```python
from build123d import *

# Parameters (mm, degrees)
F1_DEPTH       = 12
F3_D           = 5.5
F3_CSINK_D     = 12
F3_CSINK_ANGLE = 90


with BuildPart() as f1:
    # F0 (on Top) → F1 (new body)
    with BuildSketch(Plane.XY):
        with BuildLine():
            ThreePointArc((-17, 13.96424), (20.712315, -7.416198), (-22, 0))
            Line((-22, 0), (-22, 32.5))
            Line((-22, 32.5), (-32.5, 32.5))
            Line((-32.5, 32.5), (-32.5, 0))
            ThreePointArc((-32.5, 0), (-22.98097, -22.98097), (0, -32.5))
            Line((0, -32.5), (32.5, -32.5))
            Line((32.5, -32.5), (32.5, 32.5))
            Line((32.5, 32.5), (0, 32.5))
            Line((0, 32.5), (-17, 32.5))
            Line((-17, 32.5), (-17, 13.96424))
        make_face()
    extrude(amount=F1_DEPTH)

    # F3 (through all)
    with Locations(Plane(origin=(-32.5, 0, 0), x_dir=(0, -1, 0), z_dir=(-1, 0, 0))):
        with Locations((-26.5, 6)):
            CounterSinkHole(F3_D / 2, F3_CSINK_D / 2, counter_sink_angle=F3_CSINK_ANGLE)


solid = f1.part
```
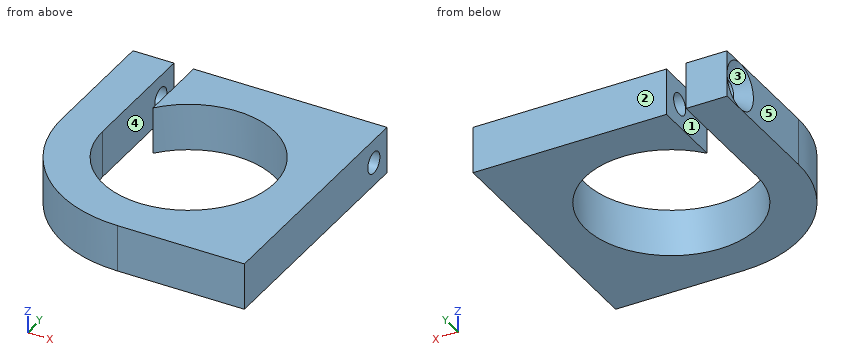
Read the model definition and answer for the solid it produces. Units are mm, in the model's axes. Face numbers are marked on the shaded views. A direction names the side the tool comes from. Coordinates: 2 decimals unless noted, no trailing zeros. Write each loop counter-clockwise with the first axis right and the second up, starting at its lowest first coordinate (ties: lowest second). Pieces come first, ordered by that corner, then holes. Notation, with made-up numbers: (-33.75, -8) -> (-28.75, -8) arc R17 ccw to (-28.75, 10) -> close; hole circle Ø10 at (71, -15). An arc over 180 degrees is marked (long way). Answer as a JSON object with one key per item and string values.
Q1. The part is cut by section B-B on y = 1.5. Give the vertices of the cut face in (x, z).
The answers:
{"outline": "(-32.5, 0) -> (-22, 0) -> (-22, 12) -> (-32.5, 12) -> close; (21.95, 0) -> (32.5, 0) -> (32.5, 12) -> (21.95, 12) -> close"}
Q2. Consider line 1 (Y direction, x = 0, z = 6.5); line 2 (Y direction, x = -1.5, z = 5.75); line 3 (Z direction, x = 1.5, y = 26.5). Determine where each line is inside the solid, lowest interval first. Write a range as [from, to].
The answers:
{"line 1": "y = [-32.5, -22], [22, 23.8], [29.2, 32.5]", "line 2": "y = [-32.47, -21.95], [21.95, 23.76], [29.24, 32.5]", "line 3": "z = [0, 3.25], [8.75, 12]"}
Q3. Determine the mould class of the marked faces 1, 2 and 3 for opening direction Y: pulls with the +Y half, pulls with the -Y half, needs draft (parallel to the pull), parting line crosses it, or undercut.
The answers:
{"face 1": "needs draft", "face 2": "pulls with the +Y half", "face 3": "undercut"}
Q4. A tool of negligible diameter and unlimited length cuts with its end or side. For the marked faces 4 and 5, from which of +Z, -Z, +X, -X, +Y, -Y can it reach the whole face along a straight path? Write none if from no direction.
The answers:
{"face 4": "+Z, -Z, +Y", "face 5": "+Z, -Z, -X, +Y, -Y"}
Q5. The part is cut by section C-C on y = 15. Give the vertices of the cut face in (x, z), then the cut area to 3 significant figures.
The answers:
{"outline": "(-32.5, 0) -> (-22, 0) -> (-22, 12) -> (-32.5, 12) -> close; (-17, 0) -> (-16.09, 0) -> (-16.09, 12) -> (-17, 12) -> close; (16.09, 0) -> (32.5, 0) -> (32.5, 12) -> (16.09, 12) -> close", "area": "334 mm2"}
Q6. The part is cut by section D-D on x = -15. Give the vertices of the cut face in (y, z), then the cut area to 3 significant figures.
The answers:
{"outline": "(-28.83, 0) -> (-16.09, 0) -> (-16.09, 12) -> (-28.83, 12) -> close; (16.09, 0) -> (32.5, 0) -> (32.5, 12) -> (16.09, 12) -> close; hole circle Ø5.5 at (26.5, 6)", "area": "326 mm2"}
Q7. Flat-ended cylindrical pins translate along their axes: pin 1 Ø4 at (y, z) = (-24.5, 9.5) entering from -X; pin 2 Ø1 at (x, z) = (-17.5, 3.5) entering from -Y; pin 3 Ø6 at (y, z) = (-20.5, 2.5) entering from -X. Find the tip coordinate at first contact, or state that the pin passes through.
The answers:
{"pin 1": "stops at x = -23.45", "pin 2": "stops at y = -27.7", "pin 3": "stops at x = -27.39"}
Q8. The part is cut by section A-A on x = 7.5. Give the vertices of the cut face in (y, z).
The answers:
{"outline": "(-32.5, 0) -> (-20.68, 0) -> (-20.68, 12) -> (-32.5, 12) -> close; (20.68, 0) -> (32.5, 0) -> (32.5, 12) -> (20.68, 12) -> close; hole circle Ø5.5 at (26.5, 6)"}
